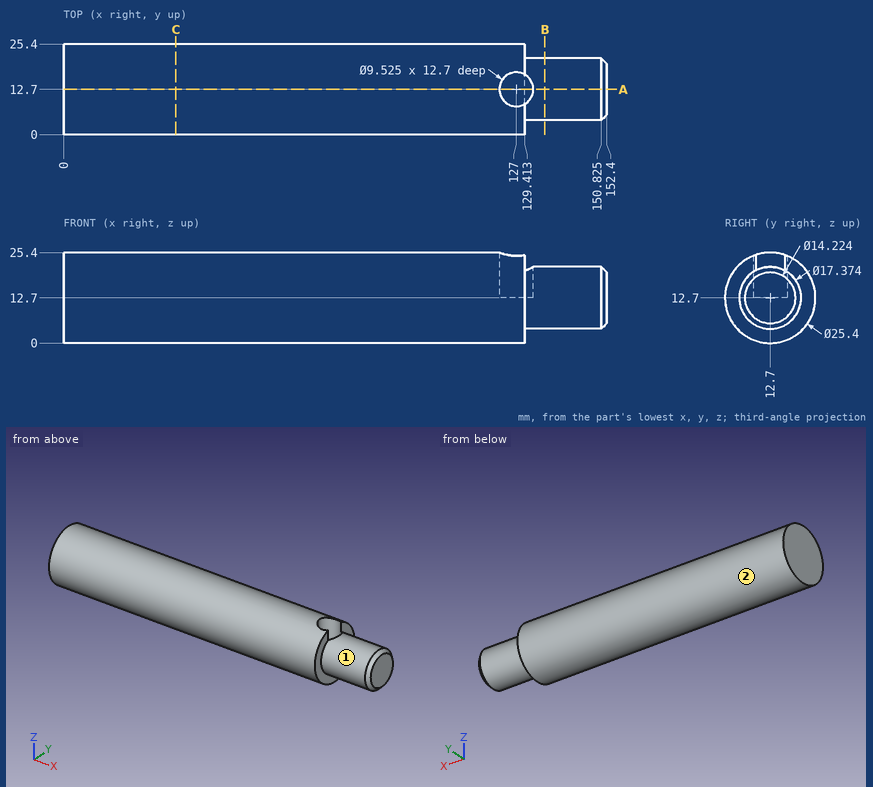
Study the drawing (mm; zero at the part's minimum x, y, z) and answer. A direction names the side the tool comes from. Round coordinates to 2 decimals unless told otherwise and drop trailing zeros. Write each loop counter-clockwise with the first axis right and the second up, starting at its lowest first coordinate (ties: lowest second). Pieces come first, ordered by that corner, then holes.
Q1. Find section C-C on x = 31.5. Determine the outline of the cut face in (y, z), and give its area (3 significant figures).
Values:
outline: circle Ø25.4 at (12.7, 12.7)
area: 507 mm2
Q2. Flat-ended cylindrical pins translate along their axes: P1, Ø1.5, axis at x = 18.5, y = 5.5, coming from the +Z side; P2, Ø1.5, axis at x = 87.5, z = 9.5, coming from the -Y side; P3, Ø1.5, axis at x = 121.5, z = 3, coming from the +Y side. Find the tip coordinate at first contact, or state that the pin passes through.
Values:
P1: stops at z = 23.64
P2: stops at y = 0.24
P3: stops at y = 21.71
Q3. A tool of negligible diameter and unlimited length cuts with its end or side. For the marked faces 1 and 2, from which of +Z, -Z, +X, -X, +Y, -Y can it reach the whole face along a straight path? Write none if from no direction.
Values:
face 1: +X
face 2: +X, -X
Q4. Find section B-B on x = 135. Determine the outline of the cut face in (y, z).
Values:
outline: circle Ø17.37 at (12.7, 12.7)
Q5. Find section A-A on y = 12.7. Determine the outline of the cut face in (x, z) (1 decimal), and give its area (3 significant figures).
Values:
outline: (0, 0) - (129.4, 0) - (129.4, 4) - (150.8, 4) - (152.4, 5.6) - (152.4, 19.8) - (150.8, 21.4) - (131.8, 21.4) - (131.8, 12.7) - (122.2, 12.7) - (122.2, 25.4) - (0, 25.4) - close
area: 3,570 mm2
Q6. Straight lines are drawn through the part: line 1 (X direction, y = 19, z = 2); line 2 (Y direction, x = 79.5, z = 12); line 3 (X direction, y = 9, z = 14). For each, find the intervals that lie inside material, in ascending order.
Values:
line 1: x = 0 to 129.41
line 2: y = 0.02 to 25.38
line 3: x = 0 to 124, 130 to 152.4
